Read the model definition and answer for the solid it produces. Units are mm, in the model's axes. A direction names the side the tool comes from. Coordinates: 2 decimals unless noted, no trailing zeros. Write each loop counter-clockwise with the first axis right and the second up, starting at its lowest first coordinate (ties: lowest second). Pieces come first, ordered by that corner, then holes.
Item 1: A tool of negligible diameter and unlimited length cuts with its end or side. For faces 4 (the face through (34.925, -776, 21)), 5 (the face through (19, -776, 0)), from which of +Z, -Z, +X, -X, +Y, -Y can it reach the whole face along a straight path? Write none if from no direction.
Item 2: Straight lines are drawn through the part: probe 1 along Z at (x, y) = (31, -1259) (3 decimals); probe 2 along X at (y, z) = (-163, 30.5) (3 decimals). For each, find the intervals that lie inside material, in ascending order.
Item 3: Determine the mould class of faces 1 (the face through (38.1, -776, 19)), 2 (the face through (16.1, -1559.15, 1.61)), 3 (the face through (15.65, -16.1, 1.61)) for opening direction Y: released by +Y, released by -Y, zero draft, split by the parting line, or undercut.
Item 4: Section A-A (y = -1377) is taken. Give the vertices of the cut face in (x, z) (3 decimals).
Item 5: Each of these flat-tipped pins is pushed along its axis until it touches: P1, Ø17.5, axis at x = 19.5, y = -1065.5, coming from the +Z side (3 decimals); P2, Ø7.5, axis at x = 15.88, y = -1540.96, coming from the -Z side. Where does it stop, or does it pass through?
Item 6: Section B-B (z = 32) is taken. Give the vertices of the cut face in (x, y) (3 decimals), then the cut area to 3 significant figures.
from build123d import *

# Parameters (mm, degrees)
F1_DEPTH = 1574.8
F3_DEPTH = 3.176
F5_D     = 8.2042


with BuildPart() as f1:
    # F0 (on Front) → F1 (new body)
    with BuildSketch(Plane.XZ):
        Polygon((0, 3.175), (0, 0), (38.1, 0), (38.1, 38.1), (34.925, 38.1), (34.925, 3.175), align=None)
    extrude(amount=F1_DEPTH)

    # F2 (on face) → F3 (cut, through all)
    with BuildSketch(Plane.XY.offset(3.175)):
        Polygon((0, -1574.8), (31.75, -1574.8), (0, -1543.05), align=None)
        Polygon((0, 0), (0, -31.75), (31.75, 0), align=None)
    extrude(amount=-F3_DEPTH, mode=Mode.SUBTRACT)

    # F5 (through all)
    with Locations(Plane.XY.offset(3.175)):
        with Locations((15.875, -1540.9644877579), (15.875, -77.9752877579)):
            Hole(F5_D / 2)


solid = f1.part
Established:
1. face 4: +Z, -X, +Y, -Y
1. face 5: -Z, +X, -X, +Y, -Y
2. probe 1: z = 0 to 3.175
2. probe 2: x = 34.925 to 38.1
3. face 1: zero draft
3. face 2: released by -Y
3. face 3: released by +Y
4. outline: (0, 0) - (38.1, 0) - (38.1, 38.1) - (34.925, 38.1) - (34.925, 3.175) - (0, 3.175) - close
5. P1: stops at z = 3.175
5. P2: passes through
6. outline: (34.925, -1574.8) - (38.1, -1574.8) - (38.1, 0) - (34.925, 0) - close
6. area: 5,000 mm2
